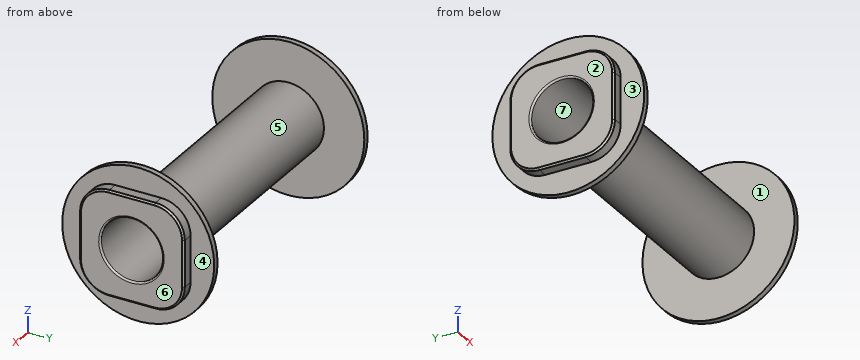
Autodesk Inventor part; units mm, degrees
ref_plane "YZ Plane" through (0, 0, 0) normal (1, 0, 0) x (0, 1, 0)
ref_plane "XZ Plane" through (0, 0, 0) normal (0, 1, 0) x (-1, 0, 0)
ref_plane "XY Plane" through (0, 0, 0) normal (0, 0, 1) x (1, 0, 0)
sketch "Skizze1" plane through (0, 0, 0) normal (0, 0, 1) x (1, 0, 0)
  line L0 (22.75, 13) -> (22.75, 5.3)
  line L1 (22.75, 5.3) -> (-22.75, 5.3)
  line L2 (-22.75, 5.3) -> (-22.75, 13)
  line L3 (-22.75, 0) -> (22.75, 0)
  line L4 (-22.75, 13) -> (-21.75, 13)
  line L5 (-21.75, 13) -> (-21.75, 6.1)
  line L6 (-21.75, 6.1) -> (21.75, 6.1)
  line L7 (21.75, 6.1) -> (21.75, 13)
  line L8 (21.75, 13) -> (22.75, 13)
  point P0 (0, 0)
  point P1 (0, 5.3)
  point P2 (0, 0)
  dimension "d0" = 10.6
  dimension "d2" = 45.5
  dimension "d8" = 1
  dimension "d9" = 0.8
  dimension "d10" = 26
revolve "Umdrehung1" add sketch "Skizze1" angle 360 about axis through (-22.75, 0, 0) along (1, 0, 0)
sketch "Skizze3" plane through (22.75, 0, 0) normal (1, 0, 0) x (0, 0, -1)
  line L0 (-8.95, -8.95) -> (8.95, -8.95)
  line L1 (8.95, -8.95) -> (8.95, 8.95)
  line L2 (8.95, 8.95) -> (-8.95, 8.95)
  line L3 (-8.95, 8.95) -> (-8.95, -8.95)
  line L4 (-8.95, -8.95) -> (8.95, 8.95) construction
  line L5 (8.95, -8.95) -> (-8.95, 8.95) construction
  circle A0 centre (0, 0) radius 5.3
  point P0 (0, 0)
  dimension "d11" = 17.9
extrude "Extrusion2" add sketch "Skizze3" along normal blind 2
fillet "Rundung2" radius 5 4 edges at (23.75, 8.95, 8.95) (23.75, 8.95, -8.95) (23.75, -8.95, 8.95) (23.75, -8.95, -8.95)
mirror "Spiegeln1" about plane through (0, 0, 0) normal (1, 0, 0) of "Extrusion2", "Rundung2"
chamfer "Fase1" distance 0.3 angle 45 4 edges at (-24.75, 0, -8.95) (-24.75, 8.95, 0) (-24.75, 0, 8.95) (-24.75, -8.95, 0)
chamfer "Fase2" distance 0.3 angle 45 4 edges at (24.75, 0, -8.95) (24.75, 8.95, 0) (24.75, 0, 8.95) (24.75, -8.95, 0)
fillet "Rundung5" radius 0.3 1 edges at (24.75, 0, 5.3)
fillet "Rundung6" radius 0.3 1 edges at (-24.75, 0, 5.3)
sketch "Skizze4" plane through (24.75, 0, 0) normal (1, 0, 0) x (0, 0, -1)
  circle A0 centre (0, 0) radius 15
  point P0 (0, 0)
ref_plane "Arbeitsebene1" through (0, 0, 0) normal (1, 0, 0) x (0, 1, 0)
properties part number "Hüllse mit Isolator" material "Nylon 6/6"
Can you work these out from the model? Positions are in its coordinate system, mm. Face numbers are marked on the shaded views. A direction names the side the tool comes from. Round coordinates to 2 decimals unless told otherwise and drop trailing zeros. Write each loop counter-clockwise with the first axis right and the second up, starting at its lowest first coordinate (ties: lowest second). Pieces come first, ordered by that corner, then holes. Notation, with made-up numbers: (-9.5, 43.5) - (46.5, 43.5) arc R23 ccw to (46.5, 73.5) - close; hole circle Ø4 at (31.25, 52). An arc over 180 degrees is marked (long way). Write each question's results on one line, items separated by ' | '. Start each with the question number.
1) Suppose I cut it at A-A (y = -10.75). List the corners of the cut face in (x, z) for me, and give its area (3 significant figures).
2) Which directions (+Z, -Z, +X, -X, +Y, -Y) give clear straight access to the entire face, cutting with the end or side of a thin tool? Please do the marked faces 1, 2, 3 and 4.
3) We'd pull the mould along Y, two halves only. Please class the marked faces 5, 6 and 7: released by +Y, released by -Y, zero draft, split by the parting line, or undercut.
4) For pin 1 Ø5 at (x, y) = (-1, 0.5) entering from -Z; pin 2 Ø1.4 at (x, y) = (-23.5, -1) entering from -Z; pin 3 Ø1.5 at (x, z) = (9.5, -3) entering from +Y, each with a flat end and sliding along its axis, tell me the tip position at first contact or that it passes through.
5) Please list where these lines run through material, in increasing order: line 1 (X direction, y = 1.75, z = -9.25); line 2 (X direction, y = -7.5, z = -5.5); line 3 (Y direction, x = -1.5, z = 3.5).
6) Suppose I cut it at B-B (x = 3). List the corners of the cut face in (y, z) for me.
Here are the results:
1) outline: (-22.75, -7.31) - (-21.75, -7.31) - (-21.75, 7.31) - (-22.75, 7.31) - close; (21.75, -7.31) - (22.75, -7.31) - (22.75, 7.31) - (21.75, 7.31) - close | area: 29.2 mm2
2) face 1: none | face 2: +Z, -Z, -X, +Y, -Y | face 3: -X | face 4: +X
3) face 5: split by the parting line | face 6: zero draft | face 7: undercut
4) pin 1: stops at z = -6.1 | pin 2: stops at z = -8.95 | pin 3: stops at y = 5.67
5) line 1: x = -22.75 to -21.75, 21.75 to 22.75 | line 2: x = -24.75 to -21.75, 21.75 to 24.75 | line 3: y = -5 to -3.98, 3.98 to 5
6) outline: circle Ø12.2 at (0, 0); hole circle Ø10.6 at (0, 0)
